Autodesk Inventor part; units mm, degrees
ref_plane "YZ Plane" through (0, 0, 0) normal (1, 0, 0) x (0, 1, 0)
ref_plane "XZ Plane" through (0, 0, 0) normal (0, 1, 0) x (-1, 0, 0)
ref_plane "XY Plane" through (0, 0, 0) normal (0, 0, 1) x (1, 0, 0)
sketch "Sketch1" plane through (0, 0, 0) normal (0, 0, 1) x (1, 0, 0)
  circle A0 centre (0, 0) radius 6.25
  line L0 (-3.2, 2.4824) -> (-3.2, -2.4824)
  line L1 (3.2, 2.4824) -> (3.2, -2.4824)
  arc A1 (3.2, 2.4824) -> (-3.2, 2.4824) centre (0, 0) ccw
  arc A2 (-3.2, -2.4824) -> (3.2, -2.4824) centre (0, 0) ccw
  dimension "d0" = 12.5
  dimension "d2" = 6.4
  dimension "d3" = 4.05
extrude "Extrusion1" add sketch "Sketch1" along normal blind 6.25
properties part number "308-05" material "Polypropylene"
Geometry check sheet. Reference: the model listing, model coordinates, mm. A direction names the side the tool comes from. Round coordinates to 2 decimals unless told otherwise and drop trailing zeros. Order: outer loops, then holes, each group sorted by start corner. A loop starts at its lowest first (then second) coordinate and runs counter-clockwise, first axis right, second up. Notation, with made-up numbers: (-12, -9) -> (30, -9) arc R26 ccw to (30, 7) -> close; hole circle Ø1 at (69, 26.25). An arc over 180 degrees is marked (long way). Return JSON: item names as keys, results as strings. Group by question number.
Q1. Material ranges on probe 1 along X at (y, z) = (-0.5, 0.5); probe 2 along Y at (x, z) = (2, 2.75); probe 3 along X at (y, z) = (3.25, 0.75), recorded low to high. Write a range as from..to.
Q2. Release check for a two-part mould opening along X. For faces 3 (the flat face through (4, 0, 6.25)), 4 (the cylindrical face through (-0.05, 4.05, 3.08)), 5 (the cylindrical face through (5.96, -1.88, 3.08)) record: released by +X, released by -X, zero draft, split by the parting line, or undercut.
Q3. Gauge pin test, flat ends, axial feed: pin 1 (1 mm diameter, centred on x = -4, z = 5, fed in from +Y); pin 2 (1.5 mm diameter, centred on y = 2, z = 3.5, fed in from -X); pin 3 (2 mm diameter, centred on x = 2.5, z = 1.5, fed in from -Y). Record the tip position at first contact, or that the pin passes through.
Q4. Section check A-A, the plane x = 0. Record the boundary of the cut face in (y, z).
Q5. Section check B-B, the plane y = 0. Record the boundary of the cut face in (x, z).
Q6. Tool access check on faces 1 (the flat face through (3.2, 0, 3)), 2 (the flat face through (4, 0, 0)). Record the directions out of +Z, -Z, +X, -X, +Y, -Y that give a thin tool (end or side, any length) a straight path to the whole face; none if there is none.
Q7. Section check D-D, the plane x = -3.5. Record the boundary of the cut face in (y, z), plus the area to 3 significant figures.
Q8. Section check C-C, the plane z = 4.75. Record the boundary of the cut face in (x, y), plus the area to 3 significant figures.
Numbers:
{
 "1": {"probe 1": "-6.23..-3.2, 3.2..6.23", "probe 2": "-5.92..-3.52, 3.52..5.92", "probe 3": "-5.34..-2.42, 2.42..5.34"},
 "2": {"face 3": "zero draft", "face 4": "undercut", "face 5": "split by the parting line"},
 "3": {"pin 1": "y = 5.18", "pin 2": "x = -6.12", "pin 3": "y = -6.07"},
 "4": {"outline": "(-6.25, 0) -> (-4.05, 0) -> (-4.05, 6.25) -> (-6.25, 6.25) -> close; (4.05, 0) -> (6.25, 0) -> (6.25, 6.25) -> (4.05, 6.25) -> close"},
 "5": {"outline": "(-6.25, 0) -> (-3.2, 0) -> (-3.2, 6.25) -> (-6.25, 6.25) -> close; (3.2, 0) -> (6.25, 0) -> (6.25, 6.25) -> (3.2, 6.25) -> close"},
 "6": {"face 1": "+Z, -Z", "face 2": "-Z, +X, -X, +Y, -Y"},
 "7": {"outline": "(-5.18, 0) -> (5.18, 0) -> (5.18, 6.25) -> (-5.18, 6.25) -> close", "area": "64.7 mm^2"},
 "8": {"outline": "circle Ø12.5 at (0, 0); hole (-3.2, -2.48) arc R4.05 ccw to (3.2, -2.48) -> (3.2, 2.48) arc R4.05 ccw to (-3.2, 2.48) -> close", "area": "76.9 mm^2"}
}
